```python
from build123d import *

# Parameters (mm, degrees)
CROQUIS1_R              = 4
CROQUIS1_R_2            = 1.5
CROQUIS1_R_3            = 3.5
CROQUIS1_R_4            = 1
SALIENTE_EXTRUIR1_DEPTH = 2
REDONDEO1_R             = 3
REDONDEO2_R             = 10
REDONDEO3_R             = 2


with BuildPart() as part:
    # Croquis1 → Saliente-Extruir1 (new body)
    with BuildSketch(Plane.XY):
        with BuildLine():
            Line((-42.426406871, 42.426406871), (-38.890872965, 45.961940777))
            Line((-38.890872965, 45.961940777), (-31.096194078, 38.16726189))
            Line((-31.096194078, 38.16726189), (-21.699105276, 28.770173088))
            ThreePointArc((-21.699105276, 28.770173088), (-18.474345963, 28.101794085), (-16.579329074, 30.795251733))
            Line((-16.579329074, 30.795251733), (-15, 80))
            Line((-15, 80), (0, 83))
            Line((0, 83), (15, 80))
            Line((15, 80), (16.579329074, 30.795251733))
            ThreePointArc((16.579329074, 30.795251733), (18.474345963, 28.101794085), (21.699105276, 28.770173088))
            Line((21.699105276, 28.770173088), (31.096194078, 38.16726189))
            Line((31.096194078, 38.16726189), (38.890872965, 45.961940777))
            Line((38.890872965, 45.961940777), (42.426406871, 42.426406871))
            Line((42.426406871, 42.426406871), (45.961940777, 38.890872965))
            Line((45.961940777, 38.890872965), (38.16726189, 31.096194078))
            Line((38.16726189, 31.096194078), (28.284271247, 21.213203436))
            ThreePointArc((28.284271247, 21.213203436), (19.497474683, 0), (28.284271247, -21.213203436))
            Line((28.284271247, -21.213203436), (38.16726189, -31.096194078))
            Line((38.16726189, -31.096194078), (45.961940777, -38.890872965))
            Line((45.961940777, -38.890872965), (42.426406871, -42.426406871))
            Line((42.426406871, -42.426406871), (38.890872965, -45.961940777))
            Line((38.890872965, -45.961940777), (31.096194078, -38.16726189))
            Line((31.096194078, -38.16726189), (21.699105276, -28.770173088))
            ThreePointArc((21.699105276, -28.770173088), (18.474345963, -28.101794085), (16.579329074, -30.795251733))
            Line((16.579329074, -30.795251733), (15, -80))
            Line((15, -80), (0, -83))
            Line((0, -83), (-15, -80))
            Line((-15, -80), (-16.579329074, -30.795251733))
            ThreePointArc((-16.579329074, -30.795251733), (-18.474345963, -28.101794085), (-21.699105276, -28.770173088))
            Line((-21.699105276, -28.770173088), (-31.096194078, -38.16726189))
            Line((-31.096194078, -38.16726189), (-38.890872965, -45.961940777))
            Line((-38.890872965, -45.961940777), (-42.426406871, -42.426406871))
            Line((-42.426406871, -42.426406871), (-45.961940777, -38.890872965))
            Line((-45.961940777, -38.890872965), (-38.16726189, -31.096194078))
            Line((-38.16726189, -31.096194078), (-28.284271247, -21.213203436))
            ThreePointArc((-28.284271247, -21.213203436), (-19.497474683, 0), (-28.284271247, 21.213203436))
            Line((-28.284271247, 21.213203436), (-38.16726189, 31.096194078))
            Line((-38.16726189, 31.096194078), (-45.961940777, 38.890872965))
            Line((-45.961940777, 38.890872965), (-42.426406871, 42.426406871))
        make_face()
        with Locations((-15.25, 15.25)):
            Circle(CROQUIS1_R, mode=Mode.SUBTRACT)
        with Locations((-24.04163056, 24.04163056)):
            Circle(CROQUIS1_R_2, mode=Mode.SUBTRACT)
        with Locations((-38.890872965, 38.890872965)):
            Circle(CROQUIS1_R_2, mode=Mode.SUBTRACT)
        with Locations(Location((38.890872965, 38.890872965, 0), (0, 0, 180))):
            Circle(CROQUIS1_R_2, mode=Mode.SUBTRACT)
        with Locations(Location((24.04163056, 24.04163056, 0), (0, 0, 180))):
            Circle(CROQUIS1_R_2, mode=Mode.SUBTRACT)
        with Locations(Location((15.25, 15.25, 0), (0, 0, 180))):
            Circle(CROQUIS1_R, mode=Mode.SUBTRACT)
        with Locations((15.25, -15.25)):
            Circle(CROQUIS1_R, mode=Mode.SUBTRACT)
        with Locations((24.04163056, -24.04163056)):
            Circle(CROQUIS1_R_2, mode=Mode.SUBTRACT)
        with Locations((38.890872965, -38.890872965)):
            Circle(CROQUIS1_R_2, mode=Mode.SUBTRACT)
        with Locations(Location((-15.25, -15.25, 0), (0, 0, 180))):
            Circle(CROQUIS1_R, mode=Mode.SUBTRACT)
        with Locations(Location((-24.04163056, -24.04163056, 0), (0, 0, 180))):
            Circle(CROQUIS1_R_2, mode=Mode.SUBTRACT)
        with Locations(Location((-38.890872965, -38.890872965, 0), (0, 0, 180))):
            Circle(CROQUIS1_R_2, mode=Mode.SUBTRACT)
        Circle(CROQUIS1_R_3, mode=Mode.SUBTRACT)
        with Locations((-11.5, -75)):
            Circle(CROQUIS1_R_2, mode=Mode.SUBTRACT)
        with Locations(Location((-14, 30, 0), (0, 0, 180))):
            Circle(CROQUIS1_R_2, mode=Mode.SUBTRACT)
        with Locations(Location((11.5, -75, 0), (0, 0, 180))):
            Circle(CROQUIS1_R_2, mode=Mode.SUBTRACT)
        with Locations((11.5, 75)):
            Circle(CROQUIS1_R_2, mode=Mode.SUBTRACT)
        with Locations(Location((-11.5, 75, 0), (0, 0, 180))):
            Circle(CROQUIS1_R_2, mode=Mode.SUBTRACT)
        with Locations((14, 30)):
            Circle(CROQUIS1_R_2, mode=Mode.SUBTRACT)
        with Locations(Location((14, -30, 0), (0, 0, 180))):
            Circle(CROQUIS1_R_2, mode=Mode.SUBTRACT)
        with Locations((-14, -30)):
            Circle(CROQUIS1_R_2, mode=Mode.SUBTRACT)
        with Locations((0, 76)):
            Circle(CROQUIS1_R_4, mode=Mode.SUBTRACT)
        with Locations(Location((0, -76, 0), (0, 0, 180))):
            Circle(CROQUIS1_R_4, mode=Mode.SUBTRACT)
        with BuildLine():
            Line((-0.620989881, -15.781703725), (-8.212878231, -22.282027547))
            ThreePointArc((-8.212878231, -22.282027547), (-8.50046857, -23.388327104), (-7.562491222, -24.04163056))
            Line((-7.562491222, -24.04163056), (8.360661842, -24.04163056))
            ThreePointArc((8.360661842, -24.04163056), (9.30628687, -23.36688939), (8.975807622, -22.253217173))
            Line((8.975807622, -22.253217173), (0.644542909, -15.75289335))
            ThreePointArc((0.644542909, -15.75289335), (0.006637615, -15.541565769), (-0.620989881, -15.781703725))
        make_face(mode=Mode.SUBTRACT)
        with BuildLine():
            Line((-7.562491222, 24.04163056), (8.360661842, 24.04163056))
            ThreePointArc((8.360661842, 24.04163056), (9.30628687, 23.36688939), (8.975807622, 22.253217173))
            Line((8.975807622, 22.253217173), (0.644542909, 15.75289335))
            ThreePointArc((0.644542909, 15.75289335), (0.006637615, 15.541565769), (-0.620989881, 15.781703725))
            Line((-0.620989881, 15.781703725), (-8.212878231, 22.282027547))
            ThreePointArc((-8.212878231, 22.282027547), (-8.50046857, 23.388327104), (-7.562491222, 24.04163056))
        make_face(mode=Mode.SUBTRACT)
        Polygon((-10, -70.668963905), (10, -70.668963905), (0, -54.625), align=None, mode=Mode.SUBTRACT)
        Polygon((0, -48.625), (-10, -32.581036095), (10, -32.581036095), align=None, mode=Mode.SUBTRACT)
        Polygon((-12.377647425, -37.01456174), (-11.479391579, -65.000149753), (-3.206987785, -51.727934965), align=None, mode=Mode.SUBTRACT)
        Polygon((3.206987785, -51.727934965), (11.479391579, -65.000149753), (12.377647425, -37.01456174), align=None, mode=Mode.SUBTRACT)
        Polygon((12.377647425, 37.01456174), (11.479391579, 65.000149753), (3.206987785, 51.727934965), align=None, mode=Mode.SUBTRACT)
        Polygon((-3.206987785, 51.727934965), (-11.479391579, 65.000149753), (-12.377647425, 37.01456174), align=None, mode=Mode.SUBTRACT)
        Polygon((-10, 32.581036095), (10, 32.581036095), (0, 48.625), align=None, mode=Mode.SUBTRACT)
        Polygon((0, 54.625), (-10, 70.668963905), (10, 70.668963905), align=None, mode=Mode.SUBTRACT)
    extrude(amount=SALIENTE_EXTRUIR1_DEPTH)

    # Redondeo1
    redondeo1_edges = [part.edges().sort_by_distance(p)[0] for p in [
        (-38.890872965, 45.961940777, 1),
        (-15, 80, 1),
        (15, 80, 1),
        (38.890872965, 45.961940777, 1),
        (45.961940777, 38.890872965, 1),
        (45.961940777, -38.890872965, 1),
        (38.890872965, -45.961940777, 1),
        (15, -80, 1),
        (-15, -80, 1),
        (-38.890872965, -45.961940777, 1),
        (-45.961940777, -38.890872965, 1),
        (-45.961940777, 38.890872965, 1),
    ]]
    fillet(redondeo1_edges, radius=REDONDEO1_R)

    # Redondeo2
    redondeo2_edges = [part.edges().sort_by_distance(p)[0] for p in [
        (0, 83, 1),
        (0, -83, 1),
    ]]
    fillet(redondeo2_edges, radius=REDONDEO2_R)

    # Redondeo3
    redondeo3_edges = [part.edges().sort_by_distance(p)[0] for p in [
        (0, -54.625, 1),
        (-10, -70.668963905, 1),
        (10, -70.668963905, 1),
        (0, -48.625, 1),
        (10, -32.581036095, 1),
        (-10, -32.581036095, 1),
        (-3.206987785, -51.727934965, 1),
        (-12.377647425, -37.01456174, 1),
        (-11.479391579, -65.000149753, 1),
        (12.377647425, -37.01456174, 1),
        (3.206987785, -51.727934965, 1),
        (11.479391579, -65.000149753, 1),
        (3.206987785, 51.727934965, 1),
        (12.377647425, 37.01456174, 1),
        (11.479391579, 65.000149753, 1),
        (-12.377647425, 37.01456174, 1),
        (-3.206987785, 51.727934965, 1),
        (-11.479391579, 65.000149753, 1),
        (0, 48.625, 1),
        (-10, 32.581036095, 1),
        (10, 32.581036095, 1),
        (0, 54.625, 1),
        (10, 70.668963905, 1),
        (-10, 70.668963905, 1),
    ]]
    fillet(redondeo3_edges, radius=REDONDEO3_R)


solid = part.part
```
Part model, mm, in its own coordinate system. A direction names the side the tool comes from. Coordinates: 2 decimals unless noted, no trailing zeros. Write each loop counter-clockwise with the first axis right and the second up, starting at its lowest first coordinate (ties: lowest second). Pieces come first, ordered by that corner, then holes.
Item 1: Slice it at B-B (y = -17.5). Write the cut outline in (x, z).
Item 2: Probe line 1 (Y direction, x = -24.5, z = 0.2); line 2 (X direction, y = 14, z = 1.5); line 3 (X direction, y = 60, z = 0.85). List the from-to ranges inside material, lowest first.
Item 3: Mould opens along Y. For faces 4 (the face through (42.407, 42.446, 0.986)), 5 (the face through (4.94, -40.7, 0.99)), 6 (the face through (-29.13, -36.2, 0.99)) say: released by +Y, released by -Y, zero draft, split by the parting line, or undercut.
Item 4: Which spindle directions (+Z, -Z, +X, -X, +Y, -Y) get a long thin tool onto all of the face, cutting with end or side? Do faces 1 (the face through (4.87, 19.05, 0.99)), 2 (the face through (29.13, 36.2, 0.99)), 3 (the face through (-42.446, 42.407, 0.986)). Say none if no direction does.
Item 5: Pin check, flat tips, straight feed: pin 1 (1 mm diameter, centred on x = -19.5, z = 0.5, fed in from -Y); pin 2 (3.5 mm diameter, centred on x = 11.5, y = -75, fed in from -Z); pin 3 (2.5 mm diameter, centred on x = 38.89, y = 38.89, fed in from +Z). Stop position of each tip, or through.
Item 6: Slice it at A-A (y = 0). Write the cut outline in (x, z), and give its area (3 significant figures).
Item 7: Slice it at C-C (z = 1.7). Count the separate pieces of the cut face and the enclosed holes in it, and give its area (3 significant figures).
Results found:
1. outline: (-25.13, 0) - (-18.56, 0) - (-18.56, 2) - (-25.13, 2) - close; (-11.94, 0) - (-2.63, 0) - (-2.63, 2) - (-11.94, 2) - close; (2.88, 0) - (11.94, 0) - (11.94, 2) - (2.88, 2) - close; (18.56, 0) - (25.13, 0) - (25.13, 2) - (18.56, 2) - close
2. line 1: y = -31.57 to -25.47, -22.61 to -16.59, 16.59 to 22.61, 25.47 to 31.57
2. line 2: x = -22.96 to -19.05, -11.45 to 11.45, 19.05 to 22.96
2. line 3: x = -15.64 to -10.82, -8.56 to -3.35, 3.35 to 8.56, 10.82 to 15.64
3. face 4: released by +Y
3. face 5: undercut
3. face 6: released by -Y
4. face 1: +Z, -Z
4. face 2: +Z, -Z, +Y
4. face 3: +Z, -Z, -X, +Y
5. pin 1: stops at y = -27.95
5. pin 2: stops at z = 0
5. pin 3: passes through
6. outline: (-19.5, 0) - (-3.5, 0) - (-3.5, 2) - (-19.5, 2) - close; (3.5, 0) - (19.5, 0) - (19.5, 2) - (3.5, 2) - close
6. area: 64.0 mm2
7. separate pieces: 1
7. enclosed holes: 33
7. area: 5,370 mm2
